For this review, take the finished solid that the model builds, in its own axes (mm). Face numbers are marked on the shaded views. A direction names the side the tool comes from. Round coordinates to 2 decimals unless told otherwise and drop trailing zeros. Loops run counter-clockwise (first coordinate to the right, second up) from the corner with the lowest first, then second, coordinate; pieces in that order, holes last.
1. Tool access review of the marked faces 3, 4 and 5: name each direction out of +Z, -Z, +X, -X, +Y, -Y from which nothing blocks a thin tool from reaching the whole face with its end or side.
2. Draft analysis for pull direction X (two halves, no side actions). For the marked faces 1 and 2, state which applies: released by +X, released by -X, zero draft, split by the parting line, or undercut.
3. To check wall thickness, follow line 1 along Y through (x, z) = (23.5, 3); line 2 along X through (y, z) = (2.55, 2.5); line 3 along Z through (x, y) = (-7, 1.65). State the ranges of each line that lie inside material, in increasing order.
4. Consider section C-C on z = 4.5. State the section outline as (x, y) points.
5. Clearance check with flat-ended pins moving along their axes: pin 1 Ø6 at (x, z) = (14.5, 4.5) entering from -Y; pin 2 Ø3.5 at (x, z) = (16, 2) entering from -Y. State where each tip first meets the part, or that it passes through.
6. Consider section B-B on y = 2.2. State how many separate pieces and enclosed holes the cut face has, then the cut area to 3 significant figures.
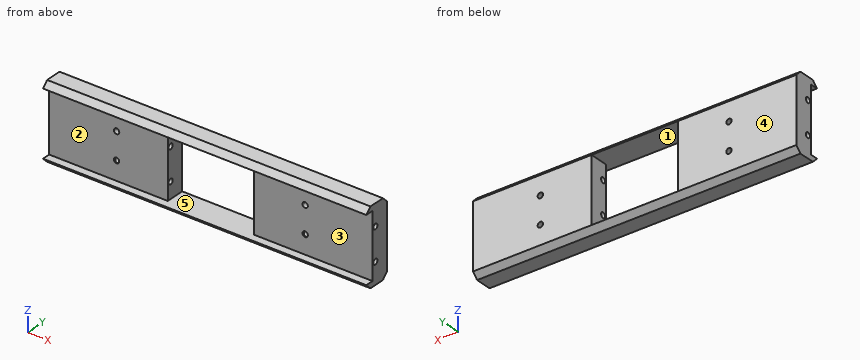
from build123d import *

# Parameters (mm, degrees)
SKETCH_1_W          = 60
SKETCH_1_H          = 14
EXTRUDE_1_DEPTH     = 5
SKETCH_2_W          = 16
SKETCH_2_H          = 12
CUT_EXTRUDE_1_DEPTH = 32.208973069
SKETCH_3_R          = 0.5
CUT_EXTRUDE_2_DEPTH = 61.613529843
SKETCH_4_W          = 22
SKETCH_4_H          = 12
CUT_EXTRUDE_3_DEPTH = 1.5
CHAMFER_1_SIZE      = 1
CHAMFER_2_SIZE      = 1
CHAMFER_3_SIZE      = 1
SKETCH_5_R          = 0.5
CUT_EXTRUDE_4_DEPTH = 32.208973069


with BuildPart() as part:
    # 草图1 → 凸台-拉伸1 (new body)
    with BuildSketch(Plane(origin=(0, 0, 0), x_dir=(1, 0, 0), z_dir=(0, 1, 0))):
        Rectangle(SKETCH_1_W, SKETCH_1_H)
    extrude(amount=EXTRUDE_1_DEPTH)

    # 草图2 → 切除-拉伸1 (cut, through all)
    with BuildSketch(Plane(origin=(0, 5, 0), x_dir=(1, 0, 0), z_dir=(0, 1, 0))):
        Rectangle(SKETCH_2_W, SKETCH_2_H)
    extrude(amount=-CUT_EXTRUDE_1_DEPTH, mode=Mode.SUBTRACT)

    # 草图3 → 切除-拉伸2 (cut, through all)
    with BuildSketch(Plane.ZY.offset(30)):
        with Locations((-3, 2.2)):
            Circle(SKETCH_3_R)
        with Locations(Location((3, 2.2, 0), (0, 0, 180))):
            Circle(SKETCH_3_R)
    extrude(amount=-CUT_EXTRUDE_2_DEPTH, mode=Mode.SUBTRACT)

    # 草图4 → 切除-拉伸3 (cut)
    with BuildSketch(Plane.XZ):
        with Locations((-19, 0)):
            Rectangle(SKETCH_4_W, SKETCH_4_H)
        with Locations((19, 0)):
            Rectangle(SKETCH_4_W, SKETCH_4_H)
    extrude(amount=-CUT_EXTRUDE_3_DEPTH, mode=Mode.SUBTRACT)

    # 倒角1
    chamfer_1_edges = [part.edges().sort_by_distance(p)[0] for p in [
        (0, 5, -7),
        (0, 5, 7),
    ]]
    chamfer(chamfer_1_edges, length=CHAMFER_1_SIZE - 0.0001)  # a hair under: the kernel refuses the full size

    # 倒角2
    chamfer_2_edges = [part.edges().sort_by_distance(p)[0] for p in [
        (0, 0, 7),
    ]]
    chamfer(chamfer_2_edges, length=CHAMFER_2_SIZE - 0.0001)  # a hair under: the kernel refuses the full size

    # 倒角3
    chamfer_3_edges = [part.edges().sort_by_distance(p)[0] for p in [
        (0, 0, -7),
    ]]
    chamfer(chamfer_3_edges, length=CHAMFER_3_SIZE - 0.0001)  # a hair under: the kernel refuses the full size

    # 草图5 → 切除-拉伸4 (cut, through all)
    with BuildSketch(Plane(origin=(0, 5, 0), x_dir=(1, 0, 0), z_dir=(0, 1, 0))):
        with Locations(Location((-17.5, 2.5, 0), (0, 0, 270))):
            Circle(SKETCH_5_R)
        with Locations(Location((17.5, 2.5, 0), (0, 0, 270))):
            Circle(SKETCH_5_R)
        with Locations(Location((17.5, -2.5, 0), (0, 0, 270))):
            Circle(SKETCH_5_R)
        with Locations(Location((-17.5, -2.5, 0), (0, 0, 90))):
            Circle(SKETCH_5_R)
    extrude(amount=-CUT_EXTRUDE_4_DEPTH, mode=Mode.SUBTRACT)


solid = part.part
Resolved:
1. face 3: +X, -X, -Y
1. face 4: +Z, -Z, +X, -X, +Y
1. face 5: -Y
2. face 1: undercut
2. face 2: zero draft
3. line 1: y = 1.5 to 1.7, 2.7 to 5
3. line 2: x = -30 to -18, -17 to -8, 8 to 17, 18 to 30
3. line 3: z = -7 to -6, 6 to 7
4. outline: (-30, 1.5) - (-8, 1.5) - (-8, 5) - (-30, 5) - close; (8, 1.5) - (30, 1.5) - (30, 5) - (8, 5) - close
5. pin 1: stops at y = 0
5. pin 2: stops at y = 1.5
6. separate pieces: 4
6. enclosed holes: 0
6. area: 558 mm2
